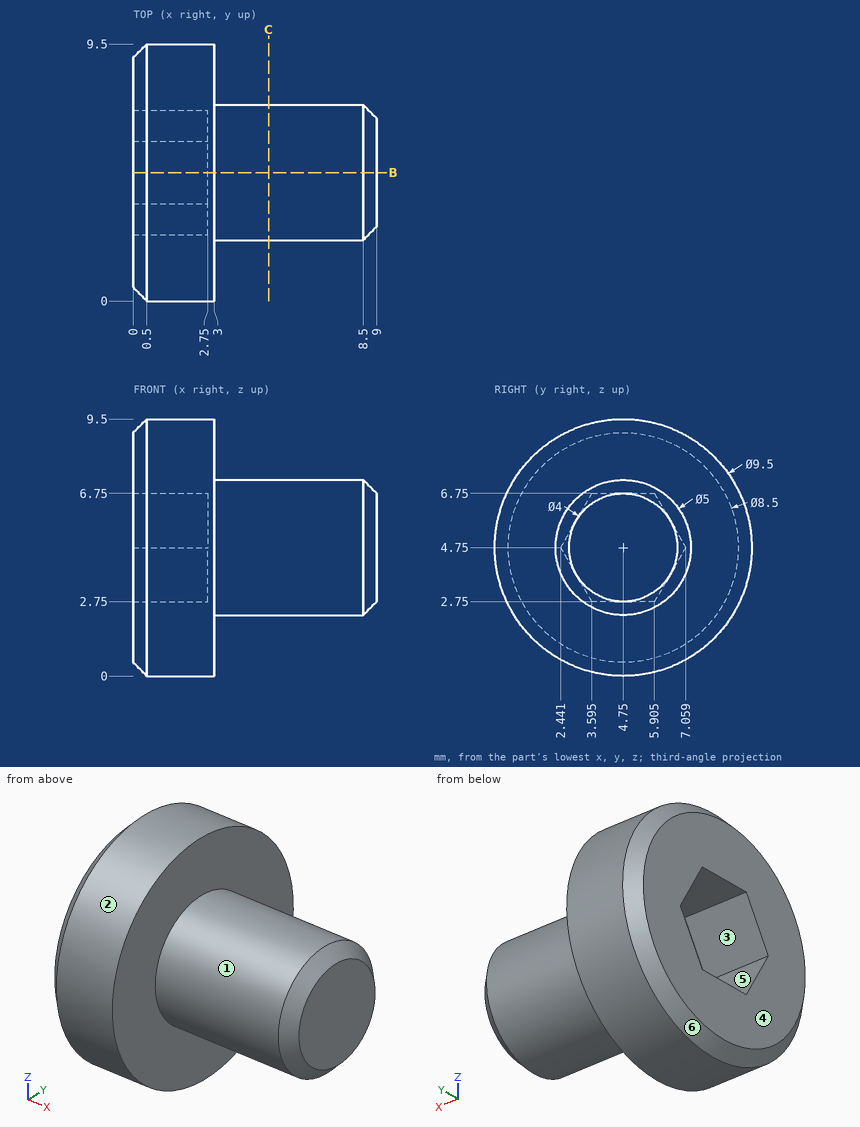
Design review of the part shown in the three views and the two pictorial views. Dimensions are in mm from the part's minimum x, y and z. A direction names the side the tool comes from. Coordinates: 2 decimals unless noted, no trailing zeros. Write each loop counter-clockwise with the first axis right and the second up, starting at its lowest first coordinate (ties: lowest second). Pieces come first, ordered by that corner, then holes. Notation, with made-up numbers: (5.5, -25.75) -> (34.5, -25.75) arc R37 cw to (34.5, 11.25) -> close; hole circle Ø5 at (22.5, 63.5). An arc over 180 degrees is marked (long way). Answer in a Markdown table with one row per item.
1. Wall thickness on probe 1 along X at (y, z) = (1.25, 5.25); probe 2 along Y at (x, z) = (2.5, 6); probe 3 along Y at (x, z) = (6.75, 6.5) (1 decimal): over which ranges is each line inside the solid? List them lowest first. Write a range as [from, to].
Answers below:
| item | result |
|---|---|
| probe 1 | x = [0, 3] |
| probe 2 | y = [0.17, 3.16], [6.34, 9.33] |
| probe 3 | y = [3, 6.5] |
2. Clearance check with flat-ended pins moving along their axes: pin 1 Ø1.5 at (x, z) = (6, 4) entering from -Y; pin 2 Ø2 at (y, z) = (5, 4.5) entering from -X; pin 3 Ø2 at (x, y) = (6, 3.5) entering from -Z. State where each tip first meets the part, or that it passes through.
Answers below:
| item | result |
|---|---|
| pin 1 | stops at y = 2.25 |
| pin 2 | stops at x = 2.75 |
| pin 3 | stops at z = 2.26 |
3. For the marked faces 1, 2 and 3, list the 3-axis set-ups (+Z, -Z, +X, -X, +Y, -Y) from which the entire face can be reached by the end or side of a thin tool; tool diameter is ignored.
Answers below:
| item | result |
|---|---|
| face 1 | +X |
| face 2 | +X, -X |
| face 3 | -X |
4. We need section C-C, the plane x = 5. State the section outline as (y, z) points, and give its area (3 significant figures).
Answers below:
| item | result |
|---|---|
| outline | circle Ø5 at (4.75, 4.75) |
| area | 19.6 mm^2 |
5. Draft analysis for pull direction Y (two halves, no side actions). For the marked faces 4, 5 and 6, state which applies: +Y half, -Y half, draft (parallel to the pull), parting line (faces both ways), or undercut.
Answers below:
| item | result |
|---|---|
| face 4 | draft |
| face 5 | undercut |
| face 6 | parting line |
6. We need section B-B, the plane y = 4.75. State the section outline as (x, z) points.
Answers below:
| item | result |
|---|---|
| outline | (0, 0.5) -> (0.5, 0) -> (3, 0) -> (3, 2.25) -> (8.5, 2.25) -> (9, 2.75) -> (9, 6.75) -> (8.5, 7.25) -> (3, 7.25) -> (3, 9.5) -> (0.5, 9.5) -> (0, 9) -> (0, 6.75) -> (2.75, 6.75) -> (2.75, 2.75) -> (0, 2.75) -> close |
